Read the model definition and answer for the solid it produces. Units are mm, in the model's axes. Face numbers are marked on the shaded views. A direction names the side the tool comes from. Give positions to 0.01 mm unless a question says otherwise; leave off trailing zeros. Order: outer loops, then holes, each group sorted by start corner. A loop starts at its lowest first (then second) coordinate and runs counter-clockwise, first axis right, second up.
Item 1: A cutting plane is placed at B-B (z = 40). Write down the section's boundary in (x, y), plus the area to 3 significant figures.
Item 2: The mould has two halves that part along X. Classify the marked faces 4, 5, 6 and 7: +X half, -X half, draft (parallel to the pull), parting line (faces both ways), or undercut.
Item 3: Find the intervals of material crossed by line 1 along Y through (x, z) = (65, -45.65); line 2 along X through (y, z) = (-22.25, -29.5); line 3 along Y through (x, z) = (-65, -45), in increasing order.
Item 4: Given pin 1 Ø6.5 at (x, y) = (65, -16.73) entering from +Z; pin 2 Ø1 at (y, z) = (-3, -15) entering from -X; pin 3 Ø6 at (y, z) = (-18, -3.5) entering from +X; pin 4 Ø12 at (y, z) = (-22.5, 26) entering from +X, each flat-ended and moving along its own axis, determine where each tip first touches the part or whether it passes through.
Item 5: A cutting plane is placed at A-A (x = -65). Write down the section's boundary in (y, z), plus the area to 3 significant figures.
Item 6: Which of the six approach directions +Z, -Z, +X, -X, +Y, -Y give full straight-line access (tool end or side, diameter ignored) to the marked faces 1, 2 and 3?
Item 7: A cutting plane is placed at C-C (x = 43). Write down the section's boundary in (y, z).
Item 8: A cutting plane is placed at D-D (x = 0). Write down the section's boundary in (y, z).
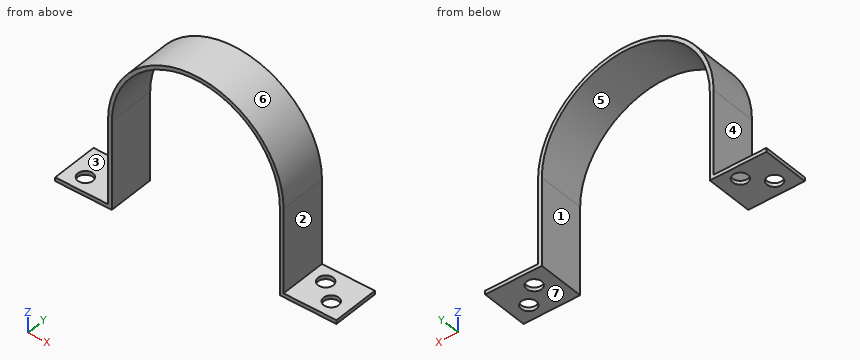
from build123d import *

# Parameters (mm, degrees)
F1_DEPTH = 25
F2_R     = 4
F3_DEPTH = 2.001


with BuildPart() as f1:
    # F0 (on Front) → F1 (new body)
    with BuildSketch(Plane.XZ):
        with BuildLine():
            ThreePointArc((-44.5, 0), (0, 44.5), (44.5, 0))
            Line((44.5, 0), (44.5, -46.5))
            Line((44.5, -46.5), (74.5, -46.5))
            Line((74.5, -46.5), (74.5, -44.5))
            Line((74.5, -44.5), (46.5, -44.5))
            Line((46.5, -44.5), (46.5, 0))
            ThreePointArc((46.5, 0), (0, 46.5), (-46.5, 0))
            Line((-46.5, 0), (-46.5, -44.5))
            Line((-46.5, -44.5), (-74.5, -44.5))
            Line((-74.5, -44.5), (-74.5, -46.5))
            Line((-74.5, -46.5), (-44.5, -46.5))
            Line((-44.5, -46.5), (-44.5, 0))
        make_face()
    extrude(amount=F1_DEPTH)

    # F2 (on face) → F3 (cut, through all)
    with BuildSketch(Plane.XY.offset(-44.5)):
        with Locations((-65, -17)):
            Circle(F2_R)
        with Locations((-55, -7)):
            Circle(F2_R)
        with Locations((55, -7.999404)):
            Circle(F2_R)
        with Locations((65, -16.7284)):
            Circle(F2_R)
    extrude(amount=-F3_DEPTH, mode=Mode.SUBTRACT)


solid = f1.part
Response values:
1. outline: (-23.71, -25) - (-19.5, -25) - (-19.5, 0) - (-23.71, 0) - close; (19.5, -25) - (23.71, -25) - (23.71, 0) - (19.5, 0) - close
1. area: 211 mm2
2. face 4: -X half
2. face 5: undercut
2. face 6: parting line
2. face 7: draft
3. line 1: y = -25 to -20.73, -12.73 to 0
3. line 2: x = -46.5 to -44.5, 44.5 to 46.5
3. line 3: y = -25 to -21, -13 to 0
4. pin 1: passes through
4. pin 2: stops at x = -46.5
4. pin 3: stops at x = 46.5
4. pin 4: stops at x = 41.98
5. outline: (-25, -46.5) - (-21, -46.5) - (-21, -44.5) - (-25, -44.5) - close; (-13, -46.5) - (0, -46.5) - (0, -44.5) - (-13, -44.5) - close
5. area: 34.0 mm2
6. face 1: -Z, +Y, -Y
6. face 2: +Z, +X, +Y, -Y
6. face 3: +Z, -X, +Y, -Y
7. outline: (-25, 11.46) - (0, 11.46) - (0, 17.7) - (-25, 17.7) - close
8. outline: (-25, 44.5) - (0, 44.5) - (0, 46.5) - (-25, 46.5) - close
